from build123d import *

# Parameters (mm, degrees)
F1_DEPTH        = 25.4
F1_COPIES_COUNT = 4


# Not quite as in the source:
# - a feature of the source that left no trace in its solid (it failed there, or was rolled back) is left out
# - a pattern or mirror of a feature is missing from the dataset's text; its kind, count and spacing are read off the source's solid


with BuildPart() as f1:
    # F0 (on Top) → F1 (new body)
    with BuildSketch(Plane.XY):
        with BuildLine():
            ThreePointArc((-11.2253201513, 11.2253201513), (-6.0750994888, 14.6665875786), (0, 15.875))
            Line((0, 15.875), (0, 101.6))
            ThreePointArc((0, 101.6), (-3.1765529485, 101.5503299422), (-6.35, 101.401368334))
            Line((-6.35, 101.401368334), (-6.35, 17.9605122421))
            ThreePointArc((-6.35, 17.9605122421), (-10.1613099439, 16.1136674976), (-13.4703841816, 13.4703841816))
            Line((-13.4703841816, 13.4703841816), (-11.2253201513, 11.2253201513))
        make_face()
    extrude(amount=F1_DEPTH)


with BuildPart() as f1_copies_1:
    # F1_copies: instance of F1
    add(f1.part.rotate(Axis((0, 0, 0), (0, 0, 1)), 1 * 360 / F1_COPIES_COUNT))


with BuildPart() as f1_copies_2:
    # F1_copies: instance of F1
    add(f1.part.rotate(Axis((0, 0, 0), (0, 0, 1)), 2 * 360 / F1_COPIES_COUNT))


with BuildPart() as f1_copies_3:
    # F1_copies: instance of F1
    add(f1.part.rotate(Axis((0, 0, 0), (0, 0, 1)), 3 * 360 / F1_COPIES_COUNT))


with BuildPart() as f1_1:
    add(f1.part)

    add(f1_copies_1.part)  # F1_copies1 merges F1_copies_1
    # F1_copies1: F1 across plane
    add(f1.part.mirror(Plane(origin=(0, 0, 0), x_dir=(0.7071067812, -0.7071067812, 0), z_dir=(-0.7071067812, -0.7071067812, 0))))



with BuildPart() as f1_2:
    add(f1_1.part)

    add(f1_copies_2.part)  # F4 merges F1_copies_2
    # F4: F1 across plane
    add(f1_1.part.mirror(Plane.XZ))



with BuildPart() as f1_3:
    add(f1_2.part)

    add(f1_copies_3.part)  # F5 merges F1_copies_3
    # F5: F1 across plane
    add(f1_2.part.mirror(Plane.YZ))


solid = f1_3.part
Source: CAD feature listing. Evaluate the final solid. Frame: model axes, mm. A direction names the side the tool comes from. Give positions to 0.01 mm unless a question says otherwise; leave off trailing zeros. Write each loop counter-clockwise with the first axis right and the second up, starting at its lowest first coordinate (ties: lowest second). Pieces come first, ordered by that corner, then holes. Notation, with made-up numbers: (45.25, 5) -> (67.25, 5) arc R10 cw to (67.25, 21) -> close; hole circle Ø8 at (69.5, -5). An arc over 180 degrees is marked (long way). Return JSON: item names as keys, results as strings. Group by question number.
1. Pin query (flat end, axial travel): pin 1 Ø12.5 at (y, z) = (-68.5, 14) entering from +X; pin 2 Ø2 at (y, z) = (-16.5, 18.5) entering from -X; pin 3 Ø5 at (x, z) = (70.5, 21) entering from +Y. Return the tip coordinate at first contact, or that it passes through.
2. Section C-C, the plane y = 69.5. Output: boundary loops of the cut face in (x, z), then the cut area to 3 significant figures.
3. Material intervals for line 1 (X direction, y = -32.5, z = 15.25); line 2 (Y direction, x = -5, z = 24), sorted ascending. Write a range as from..to.
4. Section A-A, the plane z = 11. Output: boundary loops of the cut face in (x, y) (3 decimals), then the cut area to 3 significant figures.
5. Access query for faces 1 (the face through (-60, -6.35, 13)), 2 (the face through (6.35, -60, 13)), 3 (the face through (60, 6.35, 13)), 4 (the face through (-60, 6.35, 13)). Directions: +Z, -Z, +X, -X, +Y, -Y. A direction counts if a zero-diameter tool reaches every point of the face in a straight line with its end or side. Return the directions, or none.
6. Section B-B, the plane x = 4. Output: boundary loops of the cut face in (y, z), then the cut area to 3 significant figures.
Determined:
{
 "1": {"pin 1": "stops at x = 6.35", "pin 2": "stops at x = -11.07", "pin 3": "stops at y = 6.35"},
 "2": {"outline": "(-6.35, 0) -> (6.35, 0) -> (6.35, 25.4) -> (-6.35, 25.4) -> close", "area": "323 mm2"},
 "3": {"line 1": "x = -6.35..6.35", "line 2": "y = -101.48..-15.07, 15.07..101.48"},
 "4": {"outline": "(-101.401, -6.35) -> (-17.961, -6.35) arc R19.05 ccw to (-6.35, -17.961) -> (-6.35, -101.401) arc R101.6 ccw to (6.35, -101.401) -> (6.35, -17.961) arc R19.05 ccw to (17.961, -6.35) -> (101.401, -6.35) arc R101.6 ccw to (101.401, 6.35) -> (17.961, 6.35) arc R19.05 ccw to (6.35, 17.961) -> (6.35, 101.401) arc R101.6 ccw to (-6.35, 101.401) -> (-6.35, 17.961) arc R19.05 ccw to (-17.961, 6.35) -> (-101.401, 6.35) arc R101.6 ccw to start; hole circle Ø31.75 at (0, 0)", "area": "4,560 mm2"},
 "5": {"face 1": "+Z, -Z, -X, -Y", "face 2": "+Z, -Z, +X, -Y", "face 3": "+Z, -Z, +X, +Y", "face 4": "+Z, -Z, -X, +Y"},
 "6": {"outline": "(-101.52, 0) -> (-15.36, 0) -> (-15.36, 25.4) -> (-101.52, 25.4) -> close; (15.36, 0) -> (101.52, 0) -> (101.52, 25.4) -> (15.36, 25.4) -> close", "area": "4,380 mm2"}
}
